Source: CAD feature listing. Evaluate the final solid. Frame: model axes, mm. Face numbers are marked on the shaded views. A direction names the side the tool comes from. Give positions to 0.01 mm unless a question says otherwise; leave off trailing zeros. Order: outer loops, then holes, each group sorted by start corner. A loop starts at its lowest first (then second) coordinate and runs counter-clockwise, first axis right, second up.
```python
from build123d import *

# Parameters (mm, degrees)
SKETCH_1_R          = 2.5
EXTRUDE_1_DEPTH     = 1.5
SKETCH_2_R          = 1.5
EXTRUDE_2_DEPTH     = 25
SKETCH_3_R          = 0.8
CUT_EXTRUDE_1_DEPTH = 5


with BuildPart() as part:
    # 草图1 → 凸台-拉伸1 (new body)
    with BuildSketch(Plane(origin=(0, 0, 0), x_dir=(1, 0, 0), z_dir=(0, 1, 0))):
        with Locations(Location((0, 0, 0), (0, 0, 270))):
            Circle(SKETCH_1_R)
    extrude(amount=EXTRUDE_1_DEPTH)

    # 草图2 → 凸台-拉伸2 (add)
    with BuildSketch(Plane(origin=(0, 1.5, 0), x_dir=(1, 0, 0), z_dir=(0, 1, 0))):
        with Locations(Location((0, 0, 0), (0, 0, 270))):
            Circle(SKETCH_2_R)
    extrude(amount=EXTRUDE_2_DEPTH)

    # 草图3 → 切除-拉伸1 (cut, symmetric)
    with BuildSketch(Plane.XY):
        with Locations(Location((0, 24.5, 0), (0, 0, 89.999999995))):
            Circle(SKETCH_3_R)
    extrude(amount=CUT_EXTRUDE_1_DEPTH, both=True, mode=Mode.SUBTRACT)


solid = part.part
```
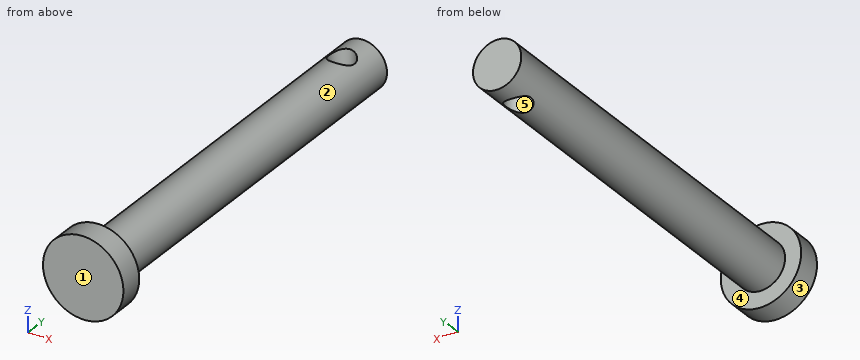
1) Pin query (flat end, axial travel): pin 1 (2 mm diameter, centred on x = 1, y = 17, fed in from -Z); pin 2 (1.5 mm diameter, centred on x = -2, y = 19.5, fed in from +Z). Return the tip coordinate at first contact, or that it passes through.
Report:
pin 1: stops at z = -1.5
pin 2: stops at z = 0.83
2) Material intervals for L1, parallel to Y at x = -2.05, z = 0.25; L2, parallel to X at y = 24.5, z = 0.3; L3, parallel to Z at x = -0.5, y = 12, sorted ascending.
Report:
L1: y = 0 to 1.5
L2: x = -1.47 to -0.8, 0.8 to 1.47
L3: z = -1.41 to 1.41
3) Section query D-D, the plane y = 14. Return the cut outline in (x, z), and give its area (3 significant figures).
Report:
outline: circle Ø3 at (0, 0)
area: 7.07 mm2
4) Section query C-C, the plane y = 24.5. Return the cut outline in (x, z).
Report:
outline: (-0.8, -1.27) - (-0.8, 1.27) arc R1.5 ccw to start; (0.8, -1.27) arc R1.5 ccw to (0.8, 1.27) - close
5) Section query B-B, the plane x = 0. Return the cut outline in (y, z).
Report:
outline: (0, -2.5) - (1.5, -2.5) - (1.5, -1.5) - (23.7, -1.5) - (23.7, 1.5) - (1.5, 1.5) - (1.5, 2.5) - (0, 2.5) - close; (25.3, -1.5) - (26.5, -1.5) - (26.5, 1.5) - (25.3, 1.5) - close
6) Reachability of the marked faces 1 and 2 from +Z, -Z, +X, -X, +Y, -Y: full face, straight path, thin tool, end or side. Return the list, or none.
Report:
face 1: +Z, -Z, +X, -X, -Y
face 2: +Y
7) Section query A-A, the plane z = 0. Return the cut outline in (x, y).
Report:
outline: (-2.5, 0) - (2.5, 0) - (2.5, 1.5) - (1.5, 1.5) - (1.5, 26.5) - (-1.5, 26.5) - (-1.5, 1.5) - (-2.5, 1.5) - close; hole circle Ø1.6 at (0, 24.5)
8) Draft query along X for the marked faces 3, 4 and 5. Return one class per face: +X half, -X half, draft (parallel to the pull), parting line (faces both ways), or undercut.
Report:
face 3: parting line
face 4: draft
face 5: undercut
